Autodesk Inventor part; units mm, degrees
ref_plane "ba2_XY" through (19.05, 7.8105, 0) normal (0, 0, 1) x (1, 0, 0)
ref_plane "ba2_YZ" through (19.05, 7.8105, 0) normal (1, 0, 0) x (0, 1, 0)
ref_plane "ba2_ZX" through (19.05, 7.8105, 0) normal (0, 1, 0) x (0, 0, 1)
sketch "Sketch_1" plane through (0, 0, 0) normal (0, 0, 1) x (1, 0, 0)
  line L0 (29.3624, 0) -> (0, 0)
  line L1 (0, 0) -> (0, 6.7691)
  line L2 (0, 6.7691) -> (0.508, 7.2771)
  line L3 (0.508, 7.2771) -> (2.7178, 7.2771)
  line L4 (2.7178, 7.2771) -> (3.3528, 6.6421)
  line L5 (3.3528, 6.6421) -> (3.9878, 6.6421)
  line L6 (3.9878, 6.6421) -> (3.9878, 7.8105)
  line L7 (3.9878, 7.8105) -> (25.3746, 7.8105)
  line L8 (25.3746, 7.8105) -> (25.3746, 6.6421)
  line L9 (25.3746, 6.6421) -> (26.0096, 6.6421)
  line L10 (26.0096, 6.6421) -> (26.6446, 7.2771)
  line L11 (26.6446, 7.2771) -> (28.8544, 7.2771)
  line L12 (28.8544, 7.2771) -> (29.3624, 6.7691)
  line L13 (29.3624, 6.7691) -> (29.3624, 0)
  line L14 (29.3624, 0) -> (0, 0)
revolve "Revolution1" add sketch "Sketch_1" angle 360 about axis through (29.3624, 0, 0) along (1, 0, 0)
sketch "Sketch2" plane through (29.3624, 0, 0) normal (1, 0, 0) x (0, 0, -1)
  point P0 (0, 0)
hole "Hole1" at (29.3624, 0, 0) direction (-1, 0, 0) diameter 5.334 depth 29.3624
sketch "Sketch_6" plane through (0, 0, 0) normal (0, 0, 1) x (1, 0, 0)
  line L0 (19.05, 0) -> (19.05, 7.8105)
  line L1 (19.05, 7.8105) -> (23.0124, 7.8105)
  line L2 (23.0124, 7.8105) -> (23.0124, 6.7945)
  line L3 (23.0124, 6.7945) -> (21.463, 6.7945)
  line L4 (21.463, 6.7945) -> (21.0337, 6.3652)
  line L5 (21.0337, 6.3652) -> (21.0337, 0)
  line L6 (21.0337, 0) -> (19.05, 0)
  line L7 (19.05, 0) -> (19.05, 7.8105)
revolve "Revolution2" cut sketch "Sketch_6" angle 360 about axis through (19.05, 0, 0) along (0, -1, 0)
thread "Thread1"
sketch "Sketch_8" plane through (0, 0, 0) normal (0, 0, 1) x (1, 0, 0)
  line L0 (29.3624, 0) -> (-29.3624, 0)
  line L1 (24.8242, 6.6421) -> (25.1116, 6.6421)
  line L2 (25.1116, 6.6421) -> (26.2128, 7.7433)
  line L3 (26.2128, 7.7433) -> (26.2128, 7.8105)
  line L4 (26.2128, 7.8105) -> (25.9926, 7.8105)
  line L5 (25.9926, 7.8105) -> (24.8242, 6.6421)
revolve "Revolution3" add sketch "Sketch_8" angle 360 about axis through (29.3624, 0, 0) along (1, 0, 0)
sketch "Sketch_14" plane through (0, 0, 0) normal (0, 0, 1) x (1, 0, 0)
  line L0 (29.3624, 0) -> (-29.3624, 0)
  line L1 (3.1496, 7.7433) -> (4.2508, 6.6421)
  line L2 (4.2508, 6.6421) -> (4.5382, 6.6421)
  line L3 (4.5382, 6.6421) -> (3.3698, 7.8105)
  line L4 (3.3698, 7.8105) -> (3.1496, 7.8105)
  line L5 (3.1496, 7.8105) -> (3.1496, 7.7433)
revolve "Revolution4" add sketch "Sketch_14" angle 360 about axis through (29.3624, 0, 0) along (1, 0, 0)
ref_plane "ba2_XY" through (19.05, 7.8105, 0) normal (0, 0, 1) x (1, 0, 0)
ref_plane "ba2_YZ" through (19.05, 7.8105, 0) normal (1, 0, 0) x (0, 1, 0)
ref_plane "ba2_ZX" through (19.05, 7.8105, 0) normal (0, 1, 0) x (0, 0, 1)
ref_plane "centar_XY" through (14.6812, 0, 0) normal (1, 0, 0) x (0, 0, -1)
ref_plane "centar_YZ" through (14.6812, 0, 0) normal (0, 0, -1) x (0, 1, 0)
ref_plane "centar_ZX" through (14.6812, 0, 0) normal (0, 1, 0) x (1, 0, 0)
ref_plane "d1_XY" through (21.463, 6.7945, 0) normal (0, 0, 1) x (1, 0, 0)
ref_plane "d1_YZ" through (21.463, 6.7945, 0) normal (1, 0, 0) x (0, 1, 0)
ref_plane "d1_ZX" through (21.463, 6.7945, 0) normal (0, 1, 0) x (0, 0, 1)
ref_plane "d2_XY" through (16.637, 6.7945, 0) normal (0, 0, 1) x (1, 0, 0)
ref_plane "d2_YZ" through (16.637, 6.7945, 0) normal (1, 0, 0) x (0, 1, 0)
ref_plane "d2_ZX" through (16.637, 6.7945, 0) normal (0, 1, 0) x (0, 0, 1)
ref_plane "to_cyl_A_XY" through (2.7178, 0, 0) normal (1, 0, 0) x (0, 0, -1)
ref_plane "to_cyl_A_YZ" through (2.7178, 0, 0) normal (0, 0, -1) x (0, 1, 0)
ref_plane "to_cyl_A_ZX" through (2.7178, 0, 0) normal (0, 1, 0) x (1, 0, 0)
ref_plane "to_cyl_B_XY" through (26.6446, 0, 0) normal (1, 0, 0) x (0, 0, -1)
ref_plane "to_cyl_B_YZ" through (26.6446, 0, 0) normal (0, 0, -1) x (0, 1, 0)
ref_plane "to_cyl_B_ZX" through (26.6446, 0, 0) normal (0, 1, 0) x (1, 0, 0)
ref_plane "to_rod_A_XY" through (29.3624, 0, 0) normal (1, 0, 0) x (0, 0, -1)
ref_plane "to_rod_A_YZ" through (29.3624, 0, 0) normal (0, 0, -1) x (0, 1, 0)
ref_plane "to_rod_A_ZX" through (29.3624, 0, 0) normal (0, 1, 0) x (1, 0, 0)
properties part number "D-68355-XP--0" material "Steel"
Check sheet for the modelled part. Datum: model origin and axes. Units: mm. A direction names the side the tool comes from. Round coordinates to 2 decimals unless told otherwise and drop trailing zeros. Write each loop counter-clockwise with the first axis right and the second up, starting at its lowest first coordinate (ties: lowest second). Pieces come first, ordered by that corner, then holes. Notation, with made-up numbers: (-27.5, -1.5) -> (-0.5, -1.5) arc R28 cw to (-0.5, 36.5) -> close; hole circle Ø10 at (61, 18.25). An arc over 180 degrees is marked (long way). Answer as CSV lines item,"result". Start each with the question number.
1) Go/stop test with flat-tipped pins: P1, Ø2, axis at x = 19, y = -1.5, coming from the +Z side; P2, Ø8, axis at x = 9, z = -6, coming from the -Y side; P3, Ø1, axis at x = 18.5, y = -2, coming from the +Z side. Record where each tip stops, or that it passes through.
2) Release check for a two-part mould opening along Z. For faces 1 (the flat face through (0, 0, -3)), 2 (the flat face through (21, 6.794, 2)), 3 (the cylindrical face through (14.831, -7.803, 0.343)) record: pulls with the +Z half, pulls with the -Z half, needs draft (parallel to the pull), parting line crosses it, or undercut.
3) Section check B-B on x = 24. Enter the section's corners in (y, z).
4) Section check A-A on x = 19.05. Enter the section's corners in (y, z).
5) Material ranges on line 1 (Y direction, x = 3.25, z = 4.5); line 2 (Y direction, x = 3.75, z = 6); line 3 (Z direction, x = 11.75, y = 0), recorded low to high. Write a range as from..to.
6) Tool access check on faces 4 (the cylindrical face through (15.09, 7.18, 0.07)), 5 (the flat face through (29.362, 0, -3)), 6 (the cylindrical face through (3.675, -1.44, -6.484)). Record the directions out of +Z, -Z, +X, -X, +Y, -Y that give a thin tool (end or side, any length) a straight path to the whole face; none if there is none.
7) Section check C-C on z = 0. State how many separate pieces and enclosed holes the cut face has, and give its area (3 significant figures).
Found:
1,P1,"stops at z = 7.79"
1,P2,"stops at y = -7.55"
1,P3,"stops at z = 7.67"
2,face 1,"needs draft"
2,face 2,"undercut"
2,face 3,"parting line crosses it"
3,outline,"circle Ø15.62 at (0, 0); hole circle Ø5.33 at (0, 0)"
4,outline,"(1.78, -1.98) arc R2.67 cw (long way) to (1.78, 1.98) -> (6.37, 1.98) -> (6.79, 2.41) -> (6.79, 3.85) arc R7.81 ccw (long way) to (6.79, -3.85) -> (6.79, -2.41) -> (6.37, -1.98) -> close"
5,line 1,"y = -6.38..-6.18, -5.02..5.02, 6.18..6.38"
5,line 2,"y = -4.38..-3.88, -2.85..2.85, 3.88..4.38"
5,line 3,"z = -7.81..-2.67, 2.67..7.81"
6,face 4,"+Y"
6,face 5,"+Z, -Z, +X, +Y, -Y"
6,face 6,"none"
7,separate pieces,"3"
7,enclosed holes,"0"
7,area,"267 mm^2"
